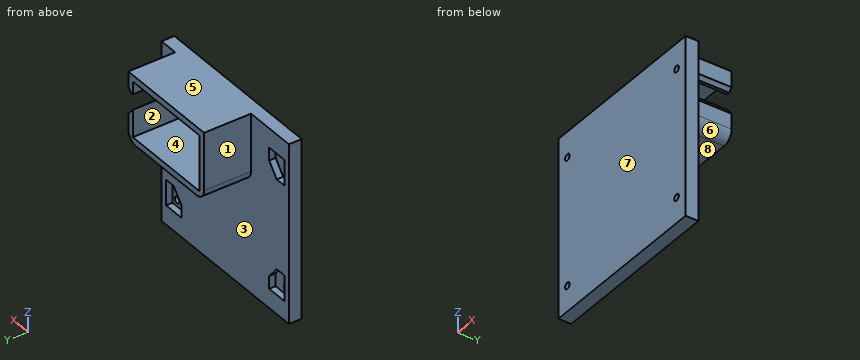
```python
from build123d import *

# Parameters (mm, degrees)
SKETCH1_W               = 84
SKETCH1_H               = 84
BOSS_EXTRUDE1_DEPTH     = 6
SKETCH2_R               = 1.5
CUT_EXTRUDE1_DEPTH      = 119.94536561
SKETCH4_R               = 1.5
CUT_EXTRUDE4_DEPTH      = 3
MIRROR3_COPY_1_SKETCH_R = 1.5
MIRROR3_COPY_1_DEPTH    = 3
SKETCH5_W               = 50
SKETCH5_H               = 32
BOSS_EXTRUDE2_DEPTH     = 22
SKETCH6_W               = 44
SKETCH6_H               = 26
CUT_EXTRUDE5_DEPTH      = 25
SKETCH8_R               = 5.5
CUT_EXTRUDE14_DEPTH     = 22
CUT_EXTRUDE15_DEPTH     = 122.396046064
FILLET2_R               = 5


with BuildPart() as part:
    # Sketch1 → Boss-Extrude1 (new body)
    with BuildSketch(Plane(origin=(0, 0, 0), x_dir=(1, 0, 0), z_dir=(0, 1, 0))):
        with Locations((42, 42)):
            Rectangle(SKETCH1_W, SKETCH1_H)
    extrude(amount=BOSS_EXTRUDE1_DEPTH)

    # Sketch2 → Cut-Extrude1 (cut, through all)
    with BuildSketch(Plane(origin=(0, 6, 0), x_dir=(1, 0, 0), z_dir=(0, 1, 0))):
        with Locations(Location((6, 72, 0), (0, 0, 270))):
            Circle(SKETCH2_R)
        with Locations(Location((6, 12, 0), (0, 0, 270))):
            Circle(SKETCH2_R)
        with Locations(Location((78, 12, 0), (0, 0, 270))):
            Circle(SKETCH2_R)
        with Locations(Location((78, 72, 0), (0, 0, 270))):
            Circle(SKETCH2_R)
    extrude(amount=-CUT_EXTRUDE1_DEPTH, mode=Mode.SUBTRACT)

    # Sketch4 → Cut-Extrude4 (cut)
    with BuildSketch(Plane(origin=(0, 6, 0), x_dir=(1, 0, 0), z_dir=(0, 1, 0))):
        Polygon((13, 15), (13, 9), (3, 9), (3, 21), (8, 21), align=None)
        with Locations(Location((6, 12, 0), (0, 0, 270))):
            Circle(SKETCH4_R, mode=Mode.SUBTRACT)
    cut_extrude4 = extrude(amount=-CUT_EXTRUDE4_DEPTH, mode=Mode.SUBTRACT)

    # Mirror2: Cut-Extrude4 across plane
    add(cut_extrude4.mirror(Plane.XY.offset(-42)), mode=Mode.SUBTRACT)

    # Mirror3: Cut-Extrude4 across plane
    add(cut_extrude4.mirror(Plane.ZY.offset(-42)), mode=Mode.SUBTRACT)

    # Mirror3 copy 1 sketch → Mirror3 copy 1 (cut)
    with BuildSketch(Plane(origin=(84, 6, -84), x_dir=(-1, 0, 0), z_dir=(0, 1, 0))):
        Polygon((13, 15), (13, 9), (3, 9), (3, 21), (8, 21), align=None)
        with Locations(Location((6, 12, 0), (0, 0, 270))):
            Circle(MIRROR3_COPY_1_SKETCH_R, mode=Mode.SUBTRACT)
    extrude(amount=-MIRROR3_COPY_1_DEPTH, mode=Mode.SUBTRACT)

    # Sketch5 → Boss-Extrude2 (add)
    with BuildSketch(Plane(origin=(0, 6, 0), x_dir=(1, 0, 0), z_dir=(0, 1, 0))):
        with Locations((50, 16)):
            Rectangle(SKETCH5_W, SKETCH5_H)
    extrude(amount=BOSS_EXTRUDE2_DEPTH)

    # Sketch6 → Cut-Extrude5 (cut)
    with BuildSketch(Plane(origin=(0, 28, 0), x_dir=(1, 0, 0), z_dir=(0, 1, 0))):
        with Locations((50, 16)):
            Rectangle(SKETCH6_W, SKETCH6_H)
    extrude(amount=-CUT_EXTRUDE5_DEPTH, mode=Mode.SUBTRACT)

    # Sketch8 → Cut-Extrude14 (cut)
    with BuildSketch(Plane(origin=(0, 28, 0), x_dir=(1, 0, 0), z_dir=(0, 1, 0))):
        with Locations((78, 12)):
            Circle(SKETCH8_R)
    extrude(amount=-CUT_EXTRUDE14_DEPTH, mode=Mode.SUBTRACT)

    # Sketch13 → Cut-Extrude15 (cut, through all)
    with BuildSketch(Plane(origin=(0, 3, 0), x_dir=(1, 0, 0), z_dir=(0, 1, 0))):
        Polygon((72, 9), (81, 9), (81, 21), (76, 21), (72, 16.2), (72, 29), (28, 29), (28, 3), (72, 3), align=None)
    extrude(amount=CUT_EXTRUDE15_DEPTH, mode=Mode.SUBTRACT)

    # Fillet2
    fillet2_edges = [part.edges().sort_by_distance(p)[0] for p in [
        (75, 17, -32),
        (25, 17, -32),
    ]]
    fillet(fillet2_edges, radius=FILLET2_R)


solid = part.part
```
The model under review builds one solid part; all positions refer to its coordinate system, in mm. Face numbers are marked on the shaded views. A direction names the side the tool comes from. Round coordinates to 2 decimals unless told otherwise and drop trailing zeros. Loops run counter-clockwise (first coordinate to the right, second up) from the corner with the lowest first, then second, coordinate; pieces in that order, holes last. Notation, with made-up numbers: M 30.5,44.5 L 49.5,44.5 A21 cw 49.5,83.5 Z; hole C -16.5,-35 d5. An arc over 180 degrees is marked long. Put each result on its own line as item: value.
Q1. Consider section B-B, the plane z = -12. Give the boundary of the cut face in (x, y).
Result set:
outline: M 0,0 L 4.5,0 L 4.5,3 L 3,3 L 3,6 L 0,6 Z; M 7.5,0 L 76.5,0 L 76.5,3 L 28,3 L 28,28 L 25,28 L 25,6 L 13,6 L 13,3 L 7.5,3 Z; M 79.5,0 L 84,0 L 84,6 L 81,6 L 81,3 L 79.5,3 Z
Q2. Machinability: for the marked faces 4, 5, 6, 7 and 8, which of the approach directions +Z, -Z, +X, -X, +Y, -Y give a long, thin tool a straight path to every point of the face, cutting with its end or side? Answer none if there is none.
Result set:
face 4: +Y
face 5: +Z, +X, -X, +Y, -Y
face 6: -Z, +X, +Y
face 7: +Z, -Z, +X, -X, -Y
face 8: -Z, +X, -X, +Y
Q3. For pin 1 (0.9 mm diameter, centred on y = 4.5, z = -70, fed in from -X); pin 2 (10 mm diameter, centred on y = 17.5, z = -21, fed in from -X); pin 3 (2 mm diameter, centred on x = 68, z = -19, fed in from +Y); pin 4 (8 mm diameter, centred on y = 13.5, z = -42, fed in from +X), all flat-tipped, find the tip position at first contact; note any pin that passes through.
Result set:
pin 1: stops at x = 0
pin 2: stops at x = 25
pin 3: stops at y = 3
pin 4: passes through
Q4. Consider section C-C, the plane y = 23.5. Give the boundary of the cut face in (x, z).
Result set:
outline: M 25,-27 A5 ccw 30,-32 L 70,-32 A5 ccw 75,-27 L 75,-19.8 L 72,-16.2 L 72,-29 L 28,-29 L 28,-3 L 72,-3 L 72,-9 L 73.39,-9 A5.5 cw 75,-7.39 L 75,0 L 25,0 Z
Q5. To check wall thickness, follow L1, parallel to Z at x = 78, y = 1.7; L2, parallel to X at y = 10.5, z = -21; L3, parallel to Z at x = 36.5, y = 17.5. State the ranges of each line that lie inside material, in increasing order.
Result set:
L1: z = -84 to -73.5, -70.5 to -13.5, -10.5 to 0
L2: x = 25 to 28, 72 to 75
L3: z = -32 to -29, -3 to 0
Q6. Mouldability with a two-part tool opening along X and no side actions: class the marked faces 1, 2 and 3 as released by +X, released by -X, zero draft, split by the parting line, or undercut.
Result set:
face 1: released by -X
face 2: undercut
face 3: zero draft
Q7. Consider section D-D, the plane z = -72. Give the boundary of the cut face in (x, y), then the cut area to 3 significant figures.
Result set:
outline: M 0,0 L 4.5,0 L 4.5,3 L 3,3 L 3,6 L 0,6 Z; M 7.5,0 L 76.5,0 L 76.5,3 L 71,3 L 71,6 L 13,6 L 13,3 L 7.5,3 Z; M 79.5,0 L 84,0 L 84,6 L 81,6 L 81,3 L 79.5,3 Z
area: 426 mm²
Q8. Consider section A-A, the plane x = 78. Give the boundary of the cut face in (y, z).
Result set:
outline: M 0,-84 L 6,-84 L 6,-75 L 3,-75 L 3,-73.5 L 0,-73.5 Z; M 0,-70.5 L 3,-70.5 L 3,-63 L 6,-63 L 6,-21 L 3,-21 L 3,-13.5 L 0,-13.5 Z; M 0,-10.5 L 3,-10.5 L 3,-9 L 6,-9 L 6,0 L 0,0 Z
